Verification items for the finished model (mm, model axes). A direction names the side the tool comes from. Give positions to 0.01 mm unless a question says otherwise; leave off trailing zeros. Order: outer loops, then holes, each group sorted by start corner. A loop starts at its lowest first (then second) coordinate and runs counter-clockwise, first axis right, second up. Notation, with made-up numbers: (-12.75, 85.5) -> (12.25, 85.5) arc R19 cw to (12.25, 101.5) -> close; hole circle Ø11 at (-27, -15). An arc over 180 degrees is marked (long way). Write each question's results on one line, items separated by ' | '. Start each with the question number.
1. Cross-section at D-D, the plane x = -21.5. Enter the section's corners in (y, z).
2. Cross-section at C-C, the plane z = 10.75. Enter the section's corners in (x, y), then the cut area to 3 significant figures.
3. Depth check by flat-ended pin: pin 1 Ø6 at (x, z) = (-33.5, 3.5) entering from +Y; pin 2 Ø3.5 at (x, y) = (-34.5, -12.5) entering from -Z; pin 3 Ø1 at (y, z) = (-37, 5.5) entering from -X. Enter the tip coordinate at first touch or a pass-through.
4. Mould release check, pull along Y, two halves, no side actions. Record for faces 4 (the face through (-45.145, -40.515, 6.108)), 5 (the face through (-35, -8.7, 10)), 6 (the face through (-25.62, -32.55, 6.25)): +Y half, -Y half, draft (parallel to the pull), parting line (faces both ways), or undercut.
5. Cross-section at A-A, the plane y = -14.7. Enter the section's corners in (x, z), then the cut area to 3 significant figures.
6. Material ranges on L1, parallel to Y at x = -40.5, z = 6; L2, parallel to Y at x = -40, z = 1.5; L3, parallel to Z at x = -34, y = -26.5, recorded low to high. Write a range as from..to.
7. Cross-section at B-B, the plane x = -47.25. Enter the section's corners in (y, z), then the cut area to 3 significant figures.
8. Set-up check for faces 1 (the face through (-27, -27.2, 6)), 2 (the face through (-40.76, -22.38, 4.32)), 3 (the face through (-36, -26, 7.548)): record each of +Z, -Z, +X, -X, +Y, -Y from which the full face is reachable in a straight line by a thin tool's end or side.
from build123d import *

# Parameters (mm, degrees)
SALIENTE_EXTRUIR2_START    = 0.2
CROQUIS2_W                 = 33
CROQUIS2_H                 = 6.1
SALIENTE_EXTRUIR2_DEPTH    = 11.8
SALIENTE_EXTRUIR3_DEPTH    = 18.5
SALIENTE_EXTRUIR5_DEPTH    = 0.4
SALIENTE_EXTRUIR6_DEPTH    = 3
CORTAR_EXTRUIR1_REACH      = 13.8
CROQUIS5_R                 = 1.75
CORTAR_EXTRUIR2_START      = -6.1
CORTAR_EXTRUIR2_DEPTH      = 2.6
CORTAR_EXTRUIR2_DEPTH_BACK = 3.5
CORTAR_EXTRUIR3_DEPTH      = 1.4
CORTAR_EXTRUIR3_DEPTH_BACK = 19.5
SALIENTE_EXTRUIR7_DEPTH    = 10.85
SALIENTE_EXTRUIR8_DEPTH    = 5
CORTAR_EXTRUIR4_DEPTH      = 35.35


with BuildPart() as part:
    # Croquis2 → Saliente-Extruir2 (new body)
    with BuildSketch(Plane.XY.offset(SALIENTE_EXTRUIR2_START)):
        with Locations((-36.15, -24.15)):
            Rectangle(CROQUIS2_W, CROQUIS2_H)
    extrude(amount=SALIENTE_EXTRUIR2_DEPTH)

    # Croquis3 → Saliente-Extruir3 (add)
    with BuildSketch(Plane.XZ.offset(27.2)):
        with BuildLine():
            Line((-42.671948935, 12), (-52.65, 12))
            Line((-52.65, 12), (-52.65, 8.2))
            Line((-52.65, 8.2), (-44.823559642, 8.2))
            ThreePointArc((-44.823559642, 8.2), (-43.981722047, 10.232475667), (-42.671948935, 12))
        make_face()
        with BuildLine():
            Line((-19.65, 12), (-29.628051065, 12))
            ThreePointArc((-29.628051065, 12), (-28.318277953, 10.232475667), (-27.476440358, 8.2))
            Line((-27.476440358, 8.2), (-19.65, 8.2))
            Line((-19.65, 8.2), (-19.65, 12))
        make_face()
        with BuildLine():
            Line((-29.628051065, 12), (-42.671948935, 12))
            ThreePointArc((-42.671948935, 12), (-43.981722047, 10.232475667), (-44.823559642, 8.2))
            Line((-44.823559642, 8.2), (-27.476440358, 8.2))
            ThreePointArc((-27.476440358, 8.2), (-28.318277953, 10.232475667), (-29.628051065, 12))
        make_face()
    extrude(amount=-SALIENTE_EXTRUIR3_DEPTH)

    # Croquis4 → Saliente-Extruir5 (add)
    with BuildSketch(Plane.XZ.offset(27.2)):
        with BuildLine():
            ThreePointArc((-27.15, 5.798050138), (-27.79244233, 9.137395851), (-29.628051065, 12))
            Line((-29.628051065, 12), (-42.671948935, 12))
            ThreePointArc((-42.671948935, 12), (-45.141099841, 6.198204681), (-43.197115342, 0.2))
            Line((-43.197115342, 0.2), (-29.102884658, 0.2))
            ThreePointArc((-29.102884658, 0.2), (-27.652234468, 2.833597245), (-27.15, 5.798050138))
        make_face()
    extrude(amount=SALIENTE_EXTRUIR5_DEPTH)

    # Croquis6 → Saliente-Extruir6 (add)
    with BuildSketch(Plane(origin=(-19.65, 0, 0), x_dir=(0, 0, -1), z_dir=(1, 0, 0))):
        Polygon((-0.2, -21.1), (-8.2, -21.1), (-8.2, -8.7), (-12, -8.7), (-12, -27.2), (-0.2, -27.2), align=None)
    extrude(amount=SALIENTE_EXTRUIR6_DEPTH)

    # Croquis5 → Cortar-Extruir1 (cut, up to next)
    with BuildSketch(Plane.XY.offset(12), mode=Mode.PRIVATE) as cortar_extruir1_sk1:
        with Locations((-22.25, -14.7)):
            Circle(CROQUIS5_R)
    cortar_extruir1_tool1 = extrude(cortar_extruir1_sk1.sketch, amount=-CORTAR_EXTRUIR1_REACH, mode=Mode.PRIVATE) & part.part
    add(cortar_extruir1_tool1.solids().sort_by_distance((-22.25, -14.7, 12))[0], mode=Mode.SUBTRACT)
    # Croquis5 → Cortar-Extruir1 (cut, up to next)
    with BuildSketch(Plane.XY.offset(12), mode=Mode.PRIVATE) as cortar_extruir1_sk2:
        with Locations((-47.25, -14.7)):
            Circle(CROQUIS5_R)
    cortar_extruir1_tool2 = extrude(cortar_extruir1_sk2.sketch, amount=-CORTAR_EXTRUIR1_REACH, mode=Mode.PRIVATE) & part.part
    add(cortar_extruir1_tool2.solids().sort_by_distance((-47.25, -14.7, 12))[0], mode=Mode.SUBTRACT)
    # Croquis5 → Cortar-Extruir1 (cut, up to next)
    with BuildSketch(Plane.XY.offset(12), mode=Mode.PRIVATE) as cortar_extruir1_sk3:
        with Locations((-46.15, -22.849986467)):
            Circle(CROQUIS5_R)
    cortar_extruir1_tool3 = extrude(cortar_extruir1_sk3.sketch, amount=-CORTAR_EXTRUIR1_REACH, mode=Mode.PRIVATE) & part.part
    add(cortar_extruir1_tool3.solids().sort_by_distance((-46.15, -22.849986, 12))[0], mode=Mode.SUBTRACT)
    # Croquis5 → Cortar-Extruir1 (cut, up to next)
    with BuildSketch(Plane.XY.offset(12), mode=Mode.PRIVATE) as cortar_extruir1_sk4:
        with Locations((-26.15, -22.849986467)):
            Circle(CROQUIS5_R)
    cortar_extruir1_tool4 = extrude(cortar_extruir1_sk4.sketch, amount=-CORTAR_EXTRUIR1_REACH, mode=Mode.PRIVATE) & part.part
    add(cortar_extruir1_tool4.solids().sort_by_distance((-26.15, -22.849986, 12))[0], mode=Mode.SUBTRACT)

    # Croquis7 → Cortar-Extruir2 (cut, two sides)
    with BuildSketch(Plane.XZ.offset(27.2).offset(CORTAR_EXTRUIR2_START)) as cortar_extruir2_sk:
        Polygon((-41.612050808, 5.798050138), (-39.88, 2.798050138), (-32.42, 2.798050138), (-30.687949192, 5.798050138), (-32.42, 8.798050138), (-39.88, 8.798050138), align=None)
    extrude(amount=CORTAR_EXTRUIR2_DEPTH, mode=Mode.SUBTRACT)
    extrude(cortar_extruir2_sk.sketch, amount=-CORTAR_EXTRUIR2_DEPTH_BACK, mode=Mode.SUBTRACT)

    # Croquis7<3> → Cortar-Extruir3 (cut, two sides)
    with BuildSketch(Plane.XZ.offset(27.2)) as cortar_extruir3_sk:
        with BuildLine():
            ThreePointArc((-37.85, 5.798050138), (-36.15, 4.098050138), (-34.45, 5.798050138))
            Line((-34.45, 5.798050138), (-37.85, 5.798050138))
        make_face()
        with BuildLine():
            Line((-37.85, 5.798050138), (-34.45, 5.798050138))
            ThreePointArc((-34.45, 5.798050138), (-36.15, 7.498050138), (-37.85, 5.798050138))
        make_face()
    extrude(amount=CORTAR_EXTRUIR3_DEPTH, mode=Mode.SUBTRACT)
    extrude(cortar_extruir3_sk.sketch, amount=-CORTAR_EXTRUIR3_DEPTH_BACK, mode=Mode.SUBTRACT)

    # Croquis8 → Saliente-Extruir7 (add)
    with BuildSketch(Plane.XZ.offset(27.2)):
        with BuildLine():
            Line((-27.219735144, 0.2), (-16.65, 0.2))
            Line((-16.65, 0.2), (-16.65, 12))
            Line((-16.65, 12), (-27.628051065, 12))
            ThreePointArc((-27.628051065, 12), (-25.616484844, 6.162541828), (-27.219735144, 0.2))
        make_face()
    extrude(amount=SALIENTE_EXTRUIR7_DEPTH)

    # Croquis9 → Saliente-Extruir8 (add)
    with BuildSketch(Plane.XZ.offset(38.05)):
        with BuildLine():
            Line((-16.65, 12), (-16.65, 0.2))
            Line((-16.65, 0.2), (-43.197115342, 0.2))
            ThreePointArc((-43.197115342, 0.2), (-45.141099841, 6.198204681), (-42.671948935, 12))
            Line((-42.671948935, 12), (-16.65, 12))
        make_face()
    extrude(amount=SALIENTE_EXTRUIR8_DEPTH)

    # Croquis10 → Cortar-Extruir4 (cut, through all)
    with BuildSketch(Plane.XZ.offset(43.05)):
        with BuildLine():
            Line((-38.15, 7.548050138), (-34.15, 7.548050138))
            ThreePointArc((-34.15, 7.548050138), (-32.4, 5.798050138), (-34.15, 4.048050138))
            Line((-34.15, 4.048050138), (-38.15, 4.048050138))
            ThreePointArc((-38.15, 4.048050138), (-39.9, 5.798050138), (-38.15, 7.548050138))
        make_face()
    extrude(amount=-CORTAR_EXTRUIR4_DEPTH, mode=Mode.SUBTRACT)


solid = part.part
Results below:
1) outline: (-43.05, 0.2) -> (-21.1, 0.2) -> (-21.1, 8.2) -> (-16.28, 8.2) -> (-16.28, 12) -> (-43.05, 12) -> close; (-13.12, 8.2) -> (-8.7, 8.2) -> (-8.7, 12) -> (-13.12, 12) -> close
2) outline: (-52.65, -27.2) -> (-43.67, -27.2) -> (-43.67, -27.6) -> (-28.63, -27.6) -> (-28.63, -27.2) -> (-26.85, -27.2) -> (-26.85, -38.05) -> (-43.67, -38.05) -> (-43.67, -43.05) -> (-16.65, -43.05) -> (-16.65, -8.7) -> (-52.65, -8.7) -> close; hole circle Ø3.5 at (-47.25, -14.7); hole circle Ø3.5 at (-46.15, -22.85); hole circle Ø3.5 at (-26.15, -22.85); hole circle Ø3.5 at (-22.25, -14.7) | area: 879 mm²
3) pin 1: stops at y = -21.1 | pin 2: stops at z = 8.2 | pin 3: stops at x = -25.64
4) face 4: draft | face 5: +Y half | face 6: undercut
5) outline: (-52.65, 8.2) -> (-49, 8.2) -> (-49, 12) -> (-52.65, 12) -> close; (-45.5, 8.2) -> (-24, 8.2) -> (-24, 12) -> (-45.5, 12) -> close; (-20.5, 8.2) -> (-16.65, 8.2) -> (-16.65, 12) -> (-20.5, 12) -> close | area: 110 mm²
6) L1: y = -43.05..-38.05, -27.6..-23.7 | L2: y = -43.05..-38.05, -27.6..-21.1 | L3: z = 0.2..4.05, 7.54..12
7) outline: (-27.2, 0.2) -> (-24.21, 0.2) -> (-24.21, 12) -> (-27.2, 12) -> close; (-21.49, 0.2) -> (-21.1, 0.2) -> (-21.1, 8.2) -> (-16.45, 8.2) -> (-16.45, 12) -> (-21.49, 12) -> close; (-12.95, 8.2) -> (-8.7, 8.2) -> (-8.7, 12) -> (-12.95, 12) -> close | area: 73.7 mm²
8) face 1: none | face 2: +Y | face 3: +Y, -Y
